Source: CAD feature listing. Evaluate the final solid. Frame: model axes, mm. A direction names the side the tool comes from. Coordinates: 2 decimals unless noted, no trailing zeros. Order: outer loops, then holes, each group sorted by start corner. A loop starts at its lowest first (then second) coordinate and runs counter-clockwise, first axis right, second up.
```python
from build123d import *

# Parameters (mm, degrees)
SKETCH_1_W          = 42.3
SKETCH_1_H          = 42.3
EXTRUDE_1_DEPTH     = 16
CHAMFER_1_SIZE      = 5
SKETCH_2_R          = 11
EXTRUDE_2_DEPTH     = 2
SKETCH_3_R          = 1.5
CUT_EXTRUDE_1_DEPTH = 5
SKETCH_4_R          = 2.5
EXTRUDE_3_DEPTH     = 10


with BuildPart() as part:
    # 草图1 → 凸台-拉伸1 (new body)
    with BuildSketch(Plane.XZ.offset(61.9)):
        Rectangle(SKETCH_1_W, SKETCH_1_H)
    extrude(amount=-EXTRUDE_1_DEPTH)

    # 倒角1
    chamfer_1_edges = [part.edges().sort_by_distance(p)[0] for p in [
        (-21.15, -53.9, -21.15),
        (-21.15, -53.9, 21.15),
        (21.15, -53.9, 21.15),
        (21.15, -53.9, -21.15),
    ]]
    chamfer(chamfer_1_edges, length=CHAMFER_1_SIZE)

    # 草图2 → 凸台-拉伸2 (add)
    with BuildSketch(Plane(origin=(0, -45.9, 0), x_dir=(-1, 0, 0), z_dir=(0, 1, 0))):
        with Locations(Location((0, 0, 0), (0, 0, 90))):
            Circle(SKETCH_2_R)
    extrude(amount=EXTRUDE_2_DEPTH)

    # 草图3 → 切除-拉伸1 (cut)
    with BuildSketch(Plane(origin=(0, -45.9, 0), x_dir=(1, 0, 0), z_dir=(0, 1, 0))):
        with Locations(Location((-15.5, 15.5, 0), (0, 0, 270))):
            Circle(SKETCH_3_R)
        with Locations(Location((15.5, 15.5, 0), (0, 0, 270))):
            Circle(SKETCH_3_R)
        with Locations(Location((15.5, -15.5, 0), (0, 0, 270))):
            Circle(SKETCH_3_R)
        with Locations(Location((-15.5, -15.5, 0), (0, 0, 270))):
            Circle(SKETCH_3_R)
    extrude(amount=-CUT_EXTRUDE_1_DEPTH, mode=Mode.SUBTRACT)

    # 草图4 → 凸台-拉伸3 (add)
    with BuildSketch(Plane(origin=(0, -43.9, 0), x_dir=(1, 0, 0), z_dir=(0, 1, 0))):
        with Locations(Location((0, 0, 0), (0, 0, 270))):
            Circle(SKETCH_4_R)
    extrude(amount=EXTRUDE_3_DEPTH)


solid = part.part
```
Q1. Material intervals for line 1 along X through (y, z) = (-47.1, 15.5); line 2 along Y through (x, z) = (16, 16); line 3 along Y through (x, z) = (-16.5, 19), sorted ascending.
Solutions:
line 1: x = -21.15 to -17, -14 to 14, 17 to 21.15
line 2: y = -61.9 to -50.9
line 3: y = -61.9 to -45.9
Q2. Set-up query: faces 1 (the flat face through (18.6, -54, 18.7)), 2 (the flat face through (-15, -50.9, -16)). Return all of +Z, -Z, +X, -X, +Y, -Y with unobstructed straight access to the full face (end or side cutting, diameter ignored); none if empty.
Solutions:
face 1: +Z, +X, +Y, -Y
face 2: +Y
Q3. Section query C-C on z = 15.5. Output: boundary loops of the cut face in (x, y).
Solutions:
outline: (-21.15, -61.9) - (21.15, -61.9) - (21.15, -45.9) - (17, -45.9) - (17, -50.9) - (14, -50.9) - (14, -45.9) - (-14, -45.9) - (-14, -50.9) - (-17, -50.9) - (-17, -45.9) - (-21.15, -45.9) - close
Q4. Section query D-D on y = -49.75. Output: boundary loops of the cut face in (x, z).
Solutions:
outline: (-21.15, -16.15) - (-16.15, -21.15) - (16.15, -21.15) - (21.15, -16.15) - (21.15, 16.15) - (16.15, 21.15) - (-16.15, 21.15) - (-21.15, 16.15) - close; hole circle Ø3 at (-15.5, -15.5); hole circle Ø3 at (-15.5, 15.5); hole circle Ø3 at (15.5, -15.5); hole circle Ø3 at (15.5, 15.5)
Q5. Pin query (flat end, axial travel): P1, Ø1.5, axis at x = 6, z = 9.5, coming from the +Y side; P2, Ø0.9, axis at x = 15.5, z = -15, coming from the +Y side; P3, Ø2, axis at x = 9.5, y = -42.5, coming from the -Z side; P4, Ø5, axis at x = -4.5, z = 16, coming from the +Y side. Return the tip coordinate at first contact, or that it passes through.
Solutions:
P1: stops at y = -43.9
P2: stops at y = -50.9
P3: passes through
P4: stops at y = -45.9
Q6. Section query B-B on y = -58.25. Output: boundary loops of the cut face in (x, z).
Solutions:
outline: (-21.15, -16.15) - (-16.15, -21.15) - (16.15, -21.15) - (21.15, -16.15) - (21.15, 16.15) - (16.15, 21.15) - (-16.15, 21.15) - (-21.15, 16.15) - close
Q7. Pull-direction query (Z, two-part tool) for faces 3 (the flat face through (16, -50.9, -16)), 4 (the flat face through (-18.6, -54, -18.7)), 5 (the flat face through (0, -61.9, 0)), 6 (the cylindrical face through (-10.74, -44.91, -2.38)); classes: pulls with the +Z half, pulls with the -Z half, needs draft (parallel to the pull), parting line crosses it, or undercut.
Solutions:
face 3: undercut
face 4: pulls with the -Z half
face 5: needs draft
face 6: parting line crosses it
Q8. Section query A-A on x = -15.5. Output: boundary loops of the cut face in (y, z), plus the area to 3 significant figures.
Solutions:
outline: (-61.9, -21.15) - (-45.9, -21.15) - (-45.9, -17) - (-50.9, -17) - (-50.9, -14) - (-45.9, -14) - (-45.9, 14) - (-50.9, 14) - (-50.9, 17) - (-45.9, 17) - (-45.9, 21.15) - (-61.9, 21.15) - close
area: 647 mm2
